```python
from build123d import *

# Parameters (mm, degrees)
BASE_FLANGE1_START = -10
BASE_FLANGE1_DEPTH = 10
CUT_EXTRUDE1_REACH = 164.687
SKETCH6_R          = 2.823671173
SKETCH6_R_2        = 2.5


# Read off the part's stored shape, not the designer's step: Base-Flange1
with BuildPart() as part:
    # Base-Flange1 outline → Base-Flange1 (new body)
    with BuildSketch(Plane.XY.offset(BASE_FLANGE1_START)):
        Polygon((50, 0), (0, 0), (0, -15), (45.980762114, -15), (139.494845224, -68.990381057), (146.994845224, -56), align=None)
    extrude(amount=BASE_FLANGE1_DEPTH)

    # Sketch6 → Cut-Extrude1 (cut, up to next)
    with BuildSketch(Plane.XY, mode=Mode.PRIVATE) as cut_extrude1_sk1:
        with Locations((10, -7.5)):
            Circle(SKETCH6_R)
    cut_extrude1_tool1 = extrude(cut_extrude1_sk1.sketch, amount=-CUT_EXTRUDE1_REACH, mode=Mode.PRIVATE) & part.part
    # Sketch6 → Cut-Extrude1 (cut, up to next)
    with BuildSketch(Plane.XY, mode=Mode.PRIVATE) as cut_extrude1_sk2:
        with Locations((134.915511346, -57.686247372)):
            Circle(SKETCH6_R_2)
    cut_extrude1_tool2 = extrude(cut_extrude1_sk2.sketch, amount=-CUT_EXTRUDE1_REACH, mode=Mode.PRIVATE) & part.part
    add(cut_extrude1_tool1.solids().sort_by_distance((10, -7.5, 0))[0], mode=Mode.SUBTRACT)
    add(cut_extrude1_tool2.solids().sort_by_distance((134.915511, -57.686247, 0))[0], mode=Mode.SUBTRACT)


solid = part.part
```
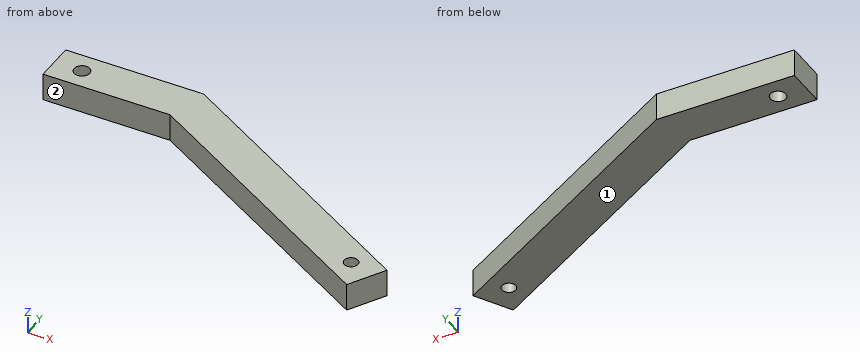
Work out the finished part from the listing and answer in its coordinate system (mm). Face numbers are marked on the shaded views. A direction names the side the tool comes from. Round coordinates to 2 decimals unless told otherwise and drop trailing zeros. Write each loop counter-clockwise with the first axis right and the second up, starting at its lowest first coordinate (ties: lowest second). Pieces come first, ordered by that corner, then holes. Notation, with made-up numbers: (61, 3.25) - (97, 3.25) arc R21 cw to (97, 33.25) - close; hole circle Ø3 at (59.25, 34). An arc over 180 degrees is marked (long way). Return JSON: item names as keys, results as strings. Group by question number.
Q1. The part is cut by section A-A on x = 10. Write down the section's boundary in (y, z), then the cut area to 3 significant figures.
Q2. For the marked faces 1 and 2, determine the directions among +Z, -Z, +X, -X, +Y, -Y from which every point of the face is accessible in a straight line to the end or side of a thin tool.
Q3. The part is cut by section B-B on y = -7.5. Write down the section's boundary in (x, z), then the cut area to 3 significant figures.
Q4. The part is cut by section D-D on x = 29. Write down the section's boundary in (y, z).
Q5. The part is cut by section C-C on z = -4. Write down the section's boundary in (x, y).
Q6. Find the intervals of material crossed by L1, parallel to Y at x = 10, z = -4.25; L2, parallel to Y at x = 7.5, z = -7.25; L3, parallel to Y at x = 44, z = -2.5, in increasing order.
Q7. Each of these flat-tipped pins is pushed along its axis until it touches: pin 1 Ø5 at (x, z) = (25, -4.5) entering from -Y; pin 2 Ø1 at (y, z) = (-18, -2.5) entering from -X; pin 3 Ø1.5 at (y, z) = (-25.5, -5.5) entering from +X. Where does it stop, or does it pass through?
Solved:
{
 "1": {"outline": "(-15, -10) - (-10.32, -10) - (-10.32, 0) - (-15, 0) - close; (-4.68, -10) - (0, -10) - (0, 0) - (-4.68, 0) - close", "area": "93.5 mm²"},
 "2": {"face 1": "-Z, +X, -X, +Y, -Y", "face 2": "+Z, -Z, -X, -Y"},
 "3": {"outline": "(0, -10) - (7.18, -10) - (7.18, 0) - (0, 0) - close; (12.82, -10) - (62.99, -10) - (62.99, 0) - (12.82, 0) - close", "area": "573 mm²"},
 "4": {"outline": "(-15, -10) - (0, -10) - (0, 0) - (-15, 0) - close"},
 "5": {"outline": "(0, -15) - (45.98, -15) - (139.49, -68.99) - (146.99, -56) - (50, 0) - (0, 0) - close; hole circle Ø5.65 at (10, -7.5); hole circle Ø5 at (134.92, -57.69)"},
 "6": {"L1": "-15 to -10.32, -4.68 to 0", "L2": "-15 to -8.81, -6.19 to 0", "L3": "-15 to 0"},
 "7": {"pin 1": "y = -15", "pin 2": "x = 50.31", "pin 3": "x = 95.47"}
}
